Read the model definition and answer for the solid it produces. Units are mm, in the model's axes. Face numbers are marked on the shaded views. A direction names the side the tool comes from. Coordinates: 2 decimals unless noted, no trailing zeros. Loops run counter-clockwise (first coordinate to the right, second up) from the corner with the lowest first, then second, coordinate; pieces in that order, holes last. Notation, with made-up numbers: M 18.5,-16.75 L 43.5,-16.75 A31 ccw 43.5,8.25 Z; hole C -37,-1 d9. An arc over 180 degrees is marked long. One line per item, written item: value. Start each with the question number.
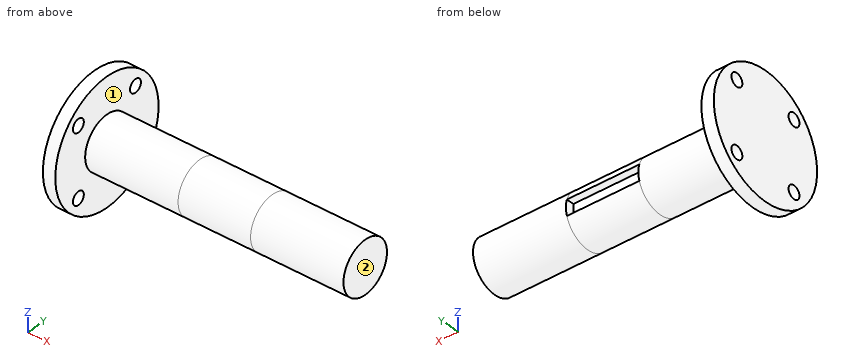
```python
from build123d import *

# Parameters (mm, degrees)
SKETCH1_R           = 8.005
BOSS_EXTRUDE1_DEPTH = 28.5
SKETCH4_R           = 19
SKETCH4_R_2         = 2
BOSS_EXTRUDE3_DEPTH = 3.8
BOSS_EXTRUDE5_DEPTH = 22.225
SKETCH7_R           = 8.005
BOSS_EXTRUDE6_DEPTH = 28.5


with BuildPart() as part:
    # Sketch1 → Boss-Extrude1 (new body)
    with BuildSketch(Plane(origin=(0, 0, 0), x_dir=(0, 0, -1), z_dir=(1, 0, 0))):
        Circle(SKETCH1_R)
    extrude(amount=BOSS_EXTRUDE1_DEPTH)

    # Sketch4 → Boss-Extrude3 (add)
    with BuildSketch(Plane.ZY):
        Circle(SKETCH4_R)
        with Locations((-10.5, 10.5)):
            Circle(SKETCH4_R_2, mode=Mode.SUBTRACT)
        with Locations((10.5, 10.5)):
            Circle(SKETCH4_R_2, mode=Mode.SUBTRACT)
        with Locations((10.5, -10.5)):
            Circle(SKETCH4_R_2, mode=Mode.SUBTRACT)
        with Locations((-10.5, -10.5)):
            Circle(SKETCH4_R_2, mode=Mode.SUBTRACT)
    extrude(amount=BOSS_EXTRUDE3_DEPTH)

    # Sketch6 → Boss-Extrude5 (add)
    with BuildSketch(Plane(origin=(28.5, 0, 0), x_dir=(0, 0, -1), z_dir=(1, 0, 0))):
        with BuildLine():
            Line((-2.3815, 5.259544), (2.3815, 5.259544))
            Line((2.3815, 5.259544), (2.3815, 7.642544))
            ThreePointArc((2.3815, 7.642544), (0, -8.005), (-2.3815, 7.642544))
            Line((-2.3815, 7.642544), (-2.3815, 5.259544))
        make_face()
    extrude(amount=BOSS_EXTRUDE5_DEPTH)

    # Sketch7 → Boss-Extrude6 (add)
    with BuildSketch(Plane(origin=(50.725, 0, 0), x_dir=(0, 0, -1), z_dir=(1, 0, 0))):
        Circle(SKETCH7_R)
    extrude(amount=BOSS_EXTRUDE6_DEPTH)


solid = part.part
```
1) Flat-ended cylindrical pins translate along their axes: pin 1 (10 mm diameter, centred on x = 43, y = 13.5, fed in from -Z); pin 2 (1.4 mm diameter, centred on x = 39, z = -0.5, fed in from +Y); pin 3 (2.5 mm diameter, centred on x = 37.5, y = 6, fed in from -Z); pin 4 (1.2 mm diameter, centred on x = 38.5, y = 6.5, fed in from +Z). Find the tip coordinate at first contact, or state that the pin passes through.
2) Section D-D (x = 2) is taken. Determine the outline of the cut face in (y, z) (3 decimals).
3) Section B-B (y = 10.5) is taken. Determine the outline of the cut face in (x, z).
4) Consider line 1 along Y through (x, z) = (-2, 10); line 2 along X through (y, z) = (-2, -15.5). Determine where each line is inside the solid, lowest interval first.
5) Section C-C (z = 0) is taken. Determine the outline of the cut face in (x, y) (3 decimals).
6) A tool of negligible diameter and unlimited length cuts with its end or side. For the marked faces 1 and 2, from which of +Z, -Z, +X, -X, +Y, -Y can it reach the whole face along a straight path? Write none if from no direction.
7) Section A-A (z = -11) is taken. Determine the outline of the cut face in (x, y), then the cut area to 3 significant figures.
Results found:
1. pin 1: passes through
1. pin 2: stops at y = 5.26
1. pin 3: stops at z = -6.44
1. pin 4: stops at z = 5.41
2. outline: C 0,0 d16.01
3. outline: M -3.8,-15.84 L 0,-15.84 L 0,-12.5 L -3.8,-12.5 Z; M -3.8,-8.5 L 0,-8.5 L 0,8.5 L -3.8,8.5 Z; M -3.8,12.5 L 0,12.5 L 0,15.84 L -3.8,15.84 Z
4. line 1: y = -16.16 to -12.44, -8.56 to 8.56, 12.44 to 16.16
4. line 2: x = -3.8 to 0
5. outline: M -3.8,-19 L 0,-19 L 0,-8.005 L 79.225,-8.005 L 79.225,8.005 L 50.725,8.005 L 50.725,5.26 L 28.5,5.26 L 28.5,8.005 L 0,8.005 L 0,19 L -3.8,19 Z
6. face 1: +X
6. face 2: +Z, -Z, +X, +Y, -Y
7. outline: M -3.8,-15.49 L 0,-15.49 L 0,-12.44 L -3.8,-12.44 Z; M -3.8,-8.56 L 0,-8.56 L 0,8.56 L -3.8,8.56 Z; M -3.8,12.44 L 0,12.44 L 0,15.49 L -3.8,15.49 Z
7. area: 88.3 mm²
